Can you work these out from the model? Positions are in its coordinate system, mm. Face numbers are marked on the shaded views. A direction names the side the tool comes from. Coordinates: 2 decimals unless noted, no trailing zeros. Order: outer loops, then holes, each group sorted by start corner. A loop starts at its lowest first (then second) coordinate and runs counter-clockwise, first axis right, second up. Notation, with made-up numbers: (6.5, -37.75) - (10.5, -37.75) arc R9 ccw to (10.5, -31.75) - close; hole circle Ø7 at (-37.5, 31.25). An arc over 180 degrees is marked (long way). Return JSON: item names as keys, results as strings. Group by question number.
1) Which directions (+Z, -Z, +X, -X, +Y, -Y) give clear straight access to the entire face, cutting with the end or side of a thin tool? Please do the marked faces 1 and 2.
2) If we mould it in two halves opening along Y, with no side actions, what happens to the marked faces 3, 4 and 5? For each: pulls with the +Y half, pulls with the -Y half, needs draft (parallel to the pull), parting line crosses it, or undercut.
3) If I drill on line 1 along Y through (x, z) = (0, 57); line 2 along Y through (x, z) = (1, 16); line 3 along X through (y, z) = (10.5, 14), over which ranges is the centre line in solid material (lowest first)?
4) Imagine slicing it at A-A (y = 0). Write out the boundary of the cut face in (x, z), and give its area (3 significant figures).
5) For pin 1 Ø12 at (x, y) = (25.5, 27.5) entering from -Z; pin 2 Ø1 at (x, z) = (5.5, 51) entering from +Y; pin 3 Ø12 at (x, z) = (27, 51.5) entering from -Y, each with a flat end and sliding along its axis, tell me the tip position at first contact or that it passes through.
6) Imagine slicing it at D-D (y = -31). Write out the boundary of the cut face in (x, z), and give its area (3 significant figures).
7) Imagine slicing it at C-C (z = 48). Write out the boundary of the cut face in (x, y).
Autodesk Fusion 360 part; units mm, degrees
cylinder "CylindrePrimitive1" add diameter 60 height 60 placed x (1, 0, 0) y (0, 1, 0) z (0, 0, 1) at (0, 0, 0)
shell "Coque1" thickness 1 removed faces 1 at (7.6631, 11.2397, 0)
cylinder "CylindrePrimitive2" add diameter 75 height 2.5 placed x (1, 0, 0) y (0, 1, 0) z (0, 0, 1) at (0, 0, 60)
hole "Perçage1" at (0, 0, 62.5) direction (0, 0, -1) diameter 59 depth 10 tip angle 118
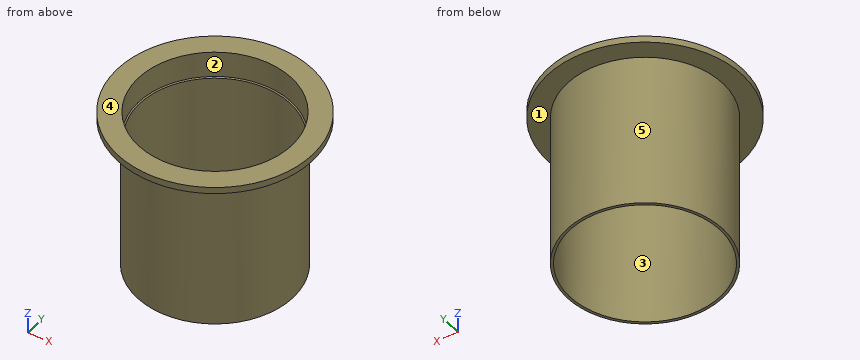
Calculated:
{
 "1": {"face 1": "-Z", "face 2": "+Z"},
 "2": {"face 3": "undercut", "face 4": "needs draft", "face 5": "parting line crosses it"},
 "3": {"line 1": "-30 to -29.5, 29.5 to 30", "line 2": "-29.98 to -28.98, 28.98 to 29.98", "line 3": "-28.1 to -27.03, 27.03 to 28.1"},
 "4": {"outline": "(-37.5, 60) - (-30, 60) - (-30, 0) - (-29, 0) - (-29, 52.2) - (-29.5, 52.5) - (-29.5, 62.5) - (-37.5, 62.5) - close; (29, 0) - (30, 0) - (30, 60) - (37.5, 60) - (37.5, 62.5) - (29.5, 62.5) - (29.5, 52.5) - (29, 52.2) - close", "area": "152 mm2"},
 "5": {"pin 1": "z = 60", "pin 2": "y = 29.58", "pin 3": "y = -21.42"},
 "6": {"outline": "(-21.1, 60) - (21.1, 60) - (21.1, 62.5) - (-21.1, 62.5) - close", "area": "106 mm2"},
 "7": {"outline": "circle Ø60 at (0, 0); hole circle Ø58 at (0, 0)"}
}
